Model file for the job. Use its own axes, mm. A direction names the side the tool comes from. Round coordinates to 2 decimals unless told otherwise and drop trailing zeros. Loops run counter-clockwise (first coordinate to the right, second up) from the corner with the lowest first, then second, coordinate; pieces in that order, holes last. Notation, with made-up numbers: (31, 87.5) -> (55, 87.5) arc R15 cw to (55, 105.5) -> close; hole circle Ø10 at (87.5, -11.5). An arc over 180 degrees is marked (long way). Use a Markdown table: item, result.
from build123d import *

# Parameters (mm, degrees)
BROCA_DE_ROSQUEAR_PARA_HELICOIDE_M2_21_D     = 2.3
BROCA_DE_ROSQUEAR_PARA_HELICOIDE_M2_21_DEPTH = 3
BROCA_DE_ROSQUEAR_PARA_HELICOIDE_M2_21_TIP   = 0.690989712


with BuildPart() as part:
    # Esboço1 → Revolução1 (revolve)
    with BuildSketch(Plane(origin=(0, 0, 0), x_dir=(0, 0, -1), z_dir=(1, 0, 0)), mode=Mode.PRIVATE) as revolu_o1_sk:
        Polygon((-15, 10), (15, 10), (15, 0), (-32, 0), (-32, 1.616532902), (-20, 1.616532902), (-20, 4.116532902), (-15, 4.116532902), align=None)
    revolve(revolu_o1_sk.sketch.rotate(Axis((0, 0, -15), (0, 0, 1)), 90), axis=Axis((0, 0, -15), (0, 0, 1)))

    # Broca de rosquear para helicoide M2.21
    with Locations(Plane.XY.offset(15)):
        with Locations((0, 6.719156642), (6.889432955, 0), (0, -6.838865025), (-7.041061835, 0)):
            Hole(BROCA_DE_ROSQUEAR_PARA_HELICOIDE_M2_21_D / 2, depth=BROCA_DE_ROSQUEAR_PARA_HELICOIDE_M2_21_DEPTH)
            with Locations((0, 0, -(BROCA_DE_ROSQUEAR_PARA_HELICOIDE_M2_21_DEPTH + BROCA_DE_ROSQUEAR_PARA_HELICOIDE_M2_21_TIP / 2))):  # 118° drill point
                Cone(0, BROCA_DE_ROSQUEAR_PARA_HELICOIDE_M2_21_D / 2, BROCA_DE_ROSQUEAR_PARA_HELICOIDE_M2_21_TIP, mode=Mode.SUBTRACT)


solid = part.part
Q1. Band-saw the part on B-B, the plane x = 5. Give the cut face in (y, z).
Results list:
| item | result |
|---|---|
| outline | (-8.66, -15) -> (8.66, -15) -> (8.66, 15) -> (-8.66, 15) -> close |
Q2. Flat gauge pins, fed straight in: pin 1 (8 mm diameter, centred on x = 5.5, y = 6.5, fed in from +Z); pin 2 (6 mm diameter, centred on x = 3, y = -4.5, fed in from +Z); pin 3 (12 mm diameter, centred on y = -8, z = 14, fed in from -X); pin 4 (4 mm diameter, centred on y = -5, z = 26, fed in from +X). Where does each tip first touch, or does it go through?
Results list:
| item | result |
|---|---|
| pin 1 | stops at z = 15 |
| pin 2 | stops at z = 20 |
| pin 3 | stops at x = -9.8 |
| pin 4 | passes through |
Q3. Tool access for faces 4 (the face through (-5.892, 0.051, 13.479)), 5 (the face through (0, 0, -15)): list every direction of +Z, -Z, +X, -X, +Y, -Y with a clear straight run to the whole face (end or side of a thin tool).
Results list:
| item | result |
|---|---|
| face 4 | +Z |
| face 5 | -Z, +X, -X, +Y, -Y |
Q4. Drill centre lines: L1, parallel to Y at x = 0, z = 13.25; L2, parallel to Z at x = -3.75, y = -4; L3, parallel to Z at x = -1.5, y = -3.5. Where is each one in solid material? Low to high. Write a range as from..to.
Results list:
| item | result |
|---|---|
| L1 | y = -10..-7.99, -5.69..5.57, 7.87..10 |
| L2 | z = -15..15 |
| L3 | z = -15..20 |
Q5. Pull direction X, two halves, no side cores. Call faces 1 (the face through (-1.9, 3.65, 17.46)), 2 (the face through (0, 0, 32)), 3 (the face through (8.04, 0.05, 13.48)): released by +X, released by -X, zero draft, split by the parting line, or undercut.
Results list:
| item | result |
|---|---|
| face 1 | split by the parting line |
| face 2 | zero draft |
| face 3 | undercut |
Q6. Band-saw the part on A-A, the plane z = 24.5. Give the cut face in (x, y), plus the area to 3 significant figures.
Results list:
| item | result |
|---|---|
| outline | circle Ø3.23 at (0, 0) |
| area | 8.21 mm² |
Q7. Band-saw the part on C-C, the plane z = 0.5. Give the cut face in (x, y).
Results list:
| item | result |
|---|---|
| outline | circle Ø20 at (0, 0) |
